Geometry: final body of the model. Coordinates: model frame, mm. A direction names the side the tool comes from. Coordinates: 2 decimals unless noted, no trailing zeros. Loops run counter-clockwise (first coordinate to the right, second up) from the corner with the lowest first, then second, coordinate; pieces in that order, holes last. Notation, with made-up numbers: (30.5, -17) -> (46.5, -17) arc R28 cw to (46.5, 7) -> close; hole circle Ø7 at (-29.75, -38.5). An arc over 180 degrees is marked (long way). One line per item, written item: value. Start each with the question number.
from build123d import *

# Parameters (mm, degrees)
F1_DEPTH      = 19.05
F0_R          = 1.9939
F2_DEPTH      = 2.54
F3_W          = 2.54
F3_H          = 1.905
F4_DEPTH      = 8.89
F5_W          = 2.54
F5_H          = 1.905
F6_DEPTH      = 11.43
F7_W          = 2.54
F7_H          = 2.54
F8_W          = 2.54
F8_H          = 2.54
F9_DEPTH      = 10.16
F10_W         = 2.54
F10_H         = 2.54
F11_DEPTH     = 11.43
F12_T1_DEPTH  = 9.525
F12_T3_DEPTH  = 14.605
F12_T5_DEPTH  = 26.035
F12_T7_DEPTH  = 9.525
F12_T9_DEPTH  = 4.445
F12_T11_DEPTH = 19.685
F12_T13_DEPTH = 22.225
F12_T15_DEPTH = 8.89
F12_T17_DEPTH = 8.89
F12_T19_DEPTH = 8.89
F12_S23_W     = 1.27
F12_S23_H     = 1.27
F12_T24_DEPTH = 1.27
F12_S29_W     = 1.27
F12_S29_H     = 1.27
F12_T30_DEPTH = 1.27


# Not quite as in the source:
# - a fillet or chamfer that OpenCascade refuses, or shapes differently, is made with other operations: its cross-section is extruded or revolved along the edge and cut away or added


with BuildPart() as f1:
    # F0 (on Front) → F1 (new body)
    with BuildSketch(Plane.XZ):
        Polygon((-23.2056408978, -6.35), (-23.2056408978, 0), (-25.7456408978, 0), (-25.7456408978, -8.89), (-9.8706408978, -8.89), (-9.8706408978, 0), (-12.4106408978, 0), (-12.4106408978, -6.35), align=None)
    extrude(amount=F1_DEPTH)

    # F0 (on Front) → F2 (join)
    with BuildSketch(Plane.XZ):
        Polygon((-25.7456408978, -8.89), (-25.7456408978, 0), (-32.0956408978, 0), (-32.0956408978, -12.7), (-3.5206408978, -12.7), (-3.5206408978, 0), (-9.8706408978, 0), (-9.8706408978, -8.89), align=None)
        Polygon((-28.6261399051, -11.2280230969), (-28.955778145, -11.2280230969), (-29.2968038878, -10.3571788012), (-30.3941995557, -10.3571788012), (-30.7310299027, -11.2280230969), (-31.0534760356, -11.2280230969), (-29.9710639241, -8.4782408335), (-29.7031579363, -8.4782408335), align=None, mode=Mode.SUBTRACT)
        with Locations((-28.2856408978, -3.81)):
            Circle(F0_R, mode=Mode.SUBTRACT)
        with Locations((-7.3306408978, -3.81)):
            Circle(F0_R, mode=Mode.SUBTRACT)
    extrude(amount=F2_DEPTH)

    # F3 (on face) → F4 (join)
    with BuildSketch(Plane.XZ.offset(19.05)):
        with Locations((-11.1406408978, -3.4925)):
            Rectangle(F3_W, F3_H)
        with Locations((-24.4756408978, -3.4925)):
            Rectangle(F3_W, F3_H)
    extrude(amount=F4_DEPTH)

    # F5 (on face) → F6 (join)
    with BuildSketch(Plane(origin=(-12.4106408978, 0, 0), x_dir=(0, -1, 0), z_dir=(-1, 0, 0))):
        with Locations((26.67, -3.4925)):
            Rectangle(F5_W, F5_H)
    extrude(amount=F6_DEPTH)

    # F7 (on face) + F8 (on face) → F9 (join)
    with BuildSketch(Plane.XY):
        with Locations((-24.4756408978, -11.43)):
            Rectangle(F7_W, F7_H)
    with BuildSketch(Plane.XY):
        with Locations((-11.1406408978, -11.43)):
            Rectangle(F8_W, F8_H)
    extrude(amount=F9_DEPTH)

    # F10 (on face) → F11 (join)
    with BuildSketch(Plane.YZ.offset(-23.2056408978)):
        with Locations((-11.43, 8.89)):
            Rectangle(F10_W, F10_H)
    extrude(amount=F11_DEPTH)

    # F12: fillet of radius 1.27 on 18 edges, made by hand

    # F12_s2 → F12_t1 (cut)
    with BuildSketch(Plane.YZ.offset(-35.2706408978)):
        with BuildLine():
            ThreePointArc((-1.27, 0), (-2.1680256121, -0.3719743879), (-2.54, -1.27))
            Line((-2.54, -1.27), (-2.54, 0))
            Line((-2.54, 0), (-1.27, 0))
        make_face()
    extrude(amount=F12_T1_DEPTH, mode=Mode.SUBTRACT)

    # F12_s4 → F12_t3 (cut)
    with BuildSketch(Plane.XY.offset(-11.43)):
        with BuildLine():
            ThreePointArc((-32.0956408978, -1.27), (-31.7236665099, -2.1680256121), (-30.8256408978, -2.54))
            Line((-30.8256408978, -2.54), (-32.0956408978, -2.54))
            Line((-32.0956408978, -2.54), (-32.0956408978, -1.27))
        make_face()
        with BuildLine():
            ThreePointArc((-3.5206408978, -1.27), (-3.8926152856, -2.1680256121), (-4.7906408978, -2.54))
            Line((-4.7906408978, -2.54), (-3.5206408978, -2.54))
            Line((-3.5206408978, -2.54), (-3.5206408978, -1.27))
        make_face()
    extrude(amount=F12_T3_DEPTH, mode=Mode.SUBTRACT)

    # F12_s6 → F12_t5 (cut)
    with BuildSketch(Plane.YZ.offset(-30.8256408978)):
        with BuildLine():
            ThreePointArc((-1.27, -12.7), (-2.1680256121, -12.3280256121), (-2.54, -11.43))
            Line((-2.54, -11.43), (-2.54, -12.7))
            Line((-2.54, -12.7), (-1.27, -12.7))
        make_face()
    extrude(amount=F12_T5_DEPTH, mode=Mode.SUBTRACT)

    # F12_s8 → F12_t7 (cut)
    with BuildSketch(Plane.YZ.offset(-9.8706408978)):
        with BuildLine():
            ThreePointArc((-1.27, 0), (-2.1680256121, -0.3719743879), (-2.54, -1.27))
            Line((-2.54, -1.27), (-2.54, 0))
            Line((-2.54, 0), (-1.27, 0))
        make_face()
    extrude(amount=F12_T7_DEPTH, mode=Mode.SUBTRACT)

    # F12_s10 → F12_t9 (cut)
    with BuildSketch(Plane.XZ.offset(-3.175)):
        with BuildLine():
            ThreePointArc((-4.7906408978, -12.7), (-3.8926152856, -12.3280256121), (-3.5206408978, -11.43))
            Line((-3.5206408978, -11.43), (-3.5206408978, -12.7))
            Line((-3.5206408978, -12.7), (-4.7906408978, -12.7))
        make_face()
        with BuildLine():
            ThreePointArc((-32.0956408978, -11.43), (-31.7236665099, -12.3280256121), (-30.8256408978, -12.7))
            Line((-30.8256408978, -12.7), (-32.0956408978, -12.7))
            Line((-32.0956408978, -12.7), (-32.0956408978, -11.43))
        make_face()
    extrude(amount=F12_T9_DEPTH, mode=Mode.SUBTRACT)

    # F12_s12 → F12_t11 (cut)
    with BuildSketch(Plane.XZ.offset(2.54)):
        with BuildLine():
            ThreePointArc((-9.8706408978, -7.62), (-10.2426152856, -8.5180256121), (-11.1406408978, -8.89))
            Line((-11.1406408978, -8.89), (-9.8706408978, -8.89))
            Line((-9.8706408978, -8.89), (-9.8706408978, -7.62))
        make_face()
        with BuildLine():
            ThreePointArc((-25.7456408978, -7.62), (-25.3736665099, -8.5180256121), (-24.4756408978, -8.89))
            Line((-24.4756408978, -8.89), (-25.7456408978, -8.89))
            Line((-25.7456408978, -8.89), (-25.7456408978, -7.62))
        make_face()
    extrude(amount=F12_T11_DEPTH, mode=Mode.SUBTRACT)

    # F12_s14 → F12_t13 (cut)
    with BuildSketch(Plane.YZ.offset(-28.9206408978)):
        with BuildLine():
            ThreePointArc((-26.67, -2.54), (-27.5680256121, -2.9119743879), (-27.94, -3.81))
            Line((-27.94, -3.81), (-27.94, -2.54))
            Line((-27.94, -2.54), (-26.67, -2.54))
        make_face()
        with BuildLine():
            ThreePointArc((-19.05, -7.62), (-18.6780256121, -8.5180256121), (-17.78, -8.89))
            Line((-17.78, -8.89), (-19.05, -8.89))
            Line((-19.05, -8.89), (-19.05, -7.62))
        make_face()
        with BuildLine():
            ThreePointArc((-27.94, -3.175), (-27.5680256121, -4.0730256121), (-26.67, -4.445))
            Line((-26.67, -4.445), (-27.94, -4.445))
            Line((-27.94, -4.445), (-27.94, -3.175))
        make_face()
        with BuildLine():
            ThreePointArc((-11.43, 10.16), (-12.3280256121, 9.7880256121), (-12.7, 8.89))
            Line((-12.7, 8.89), (-12.7, 10.16))
            Line((-12.7, 10.16), (-11.43, 10.16))
        make_face()
        with BuildLine():
            ThreePointArc((-10.16, 8.89), (-10.5319743879, 9.7880256121), (-11.43, 10.16))
            Line((-11.43, 10.16), (-10.16, 10.16))
            Line((-10.16, 10.16), (-10.16, 8.89))
        make_face()
    extrude(amount=F12_T13_DEPTH, mode=Mode.SUBTRACT)

    # F12_s16 → F12_t15 (cut)
    with BuildSketch(Plane.YZ.offset(-28.9206408978)):
        with BuildLine():
            ThreePointArc((-19.05, -1.27), (-18.6780256121, -0.3719743879), (-17.78, 0))
            Line((-17.78, 0), (-19.05, 0))
            Line((-19.05, 0), (-19.05, -1.27))
        make_face()
    extrude(amount=F12_T15_DEPTH, mode=Mode.SUBTRACT)

    # F12_s18 → F12_t17 (cut)
    with BuildSketch(Plane.YZ.offset(-15.5856408978)):
        with BuildLine():
            ThreePointArc((-17.78, 0), (-18.6780256121, -0.3719743879), (-19.05, -1.27))
            Line((-19.05, -1.27), (-19.05, 0))
            Line((-19.05, 0), (-17.78, 0))
        make_face()
    extrude(amount=F12_T17_DEPTH, mode=Mode.SUBTRACT)

    # F12_s20 → F12_t19 (cut)
    with BuildSketch(Plane.XZ.offset(6.985)):
        with BuildLine():
            ThreePointArc((-25.7456408978, 8.89), (-25.3736665099, 9.7880256121), (-24.4756408978, 10.16))
            Line((-24.4756408978, 10.16), (-25.7456408978, 10.16))
            Line((-25.7456408978, 10.16), (-25.7456408978, 8.89))
        make_face()
        with BuildLine():
            ThreePointArc((-9.8706408978, 8.89), (-10.2426152856, 9.7880256121), (-11.1406408978, 10.16))
            Line((-11.1406408978, 10.16), (-9.8706408978, 10.16))
            Line((-9.8706408978, 10.16), (-9.8706408978, 8.89))
        make_face()
    extrude(amount=F12_T19_DEPTH, mode=Mode.SUBTRACT)


with BuildPart() as f12_tool22:
    # F12_s23 → F12_t24 (new body)
    with BuildSketch(Plane.YZ.offset(-30.8256408978)):
        with Locations((-1.905, -12.065)):
            Rectangle(F12_S23_W, F12_S23_H)
    extrude(amount=-F12_T24_DEPTH)

    # F12_s25 → F12_t26 (revolve, cut)
    with BuildSketch(Plane(origin=(-30.8256408978, -1.27, -11.43), x_dir=(0, 0.7071067812, 0.7071067812), z_dir=(0, -0.7071067812, 0.7071067812))):
        with BuildLine():
            ThreePointArc((0, -1.27), (1.27, 0), (0, 1.27))
            Line((0, 1.27), (0, -1.27))
        make_face()
    revolve(axis=Axis((-30.8256408978, -1.27, -11.43), (-1, 0, 0)), mode=Mode.SUBTRACT)


with BuildPart() as f1_1:
    add(f1.part)

    # F12_t21: cut F12_tool22
    add(f12_tool22.part, mode=Mode.SUBTRACT)


with BuildPart() as f12_tool28:
    # F12_s29 → F12_t30 (new body)
    with BuildSketch(Plane.YZ.offset(-4.7906408978)):
        with Locations((-1.905, -12.065)):
            Rectangle(F12_S29_W, F12_S29_H)
    extrude(amount=F12_T30_DEPTH)

    # F12_s31 → F12_t32 (revolve, cut)
    with BuildSketch(Plane(origin=(-4.7906408978, -1.27, -11.43), x_dir=(0, 0.7071067812, 0.7071067812), z_dir=(0, 0.7071067812, -0.7071067812))):
        with BuildLine():
            ThreePointArc((0, -1.27), (1.27, 0), (0, 1.27))
            Line((0, 1.27), (0, -1.27))
        make_face()
    revolve(axis=Axis((-4.7906408978, -1.27, -11.43), (1, 0, 0)), mode=Mode.SUBTRACT)


with BuildPart() as f1_2:
    add(f1_1.part)

    # F12_t27: cut F12_tool28
    add(f12_tool28.part, mode=Mode.SUBTRACT)


solid = f1_2.part
1. Section A-A on z = 2.75. Return the cut outline in (x, y), plus the area to 3 significant figures.
2. Pin query (flat end, axial travel): pin 1 Ø2.5 at (x, z) = (-15.5, -6.5) entering from -Y; pin 2 Ø7 at (x, y) = (-7.5, -5) entering from +Z; pin 3 Ø4 at (x, y) = (-7, -19.5) entering from +Z (3 decimals); pin 4 Ø2 at (x, y) = (-24, -16.5) entering from -Z. Return the tip coordinate at first contact, or that it passes through.
3. Draft query along Z for faces 4 (the face through (-16, -26, -2.54)), 5 (the face through (-3.903, -0.626, -12.338)), 6 (the face through (-18, -25.4, -4)), 7 (the face through (-29.172, -1.252, -9.834)). Return one class per face: released by +Z, released by -Z, zero draft, split by the parting line, or undercut.
4. Section C-C on y = -14.25. Return the cut outline in (x, z).
5. Line query: L1, parallel to X at y = -11.25, z = 6.25; L2, parallel to Y at x = -8.25, z = -9.5; L3, parallel to Y at x = -18.25, z = -7. Output: solid intervals per line, ascending. Write a range as [from, to].
6. Section B-B on x = -18. Count the separate pieces of the cut face and the enclosed holes in it, plus the area to 3 significant figures.
7. Set-up query: faces 1 (the face through (-23.206, -13, -3)), 2 (the face through (-29.124, -1.252, -10.799)), 3 (the face through (-10.233, -10.679, -8.508)). Return all of +Z, -Z, +X, -X, +Y, -Y with unobstructed straight access to the full face (end or side cutting, diameter ignored); none if empty.
8. Section D-D on y = -11. Return the cut outline in (x, z), plus the area to 3 significant figures.
Checks:
1. outline: (-25.75, -12.7) -> (-23.21, -12.7) -> (-23.21, -10.16) -> (-25.75, -10.16) -> close; (-12.41, -12.7) -> (-9.87, -12.7) -> (-9.87, -10.16) -> (-12.41, -10.16) -> close
1. area: 12.9 mm²
2. pin 1: y = -19.05
2. pin 2: z = 0
2. pin 3: through
2. pin 4: z = -8.89
3. face 4: released by +Z
3. face 5: released by -Z
3. face 6: zero draft
3. face 7: undercut
4. outline: (-25.75, -7.62) arc R1.27 ccw to (-24.48, -8.89) -> (-11.14, -8.89) arc R1.27 ccw to (-9.87, -7.62) -> (-9.87, 0) -> (-12.41, 0) -> (-12.41, -6.35) -> (-23.21, -6.35) -> (-23.21, 0) -> (-25.75, 0) -> close
5. L1: [-25.75, -23.21], [-12.41, -9.87]
5. L2: [-2.54, 0]
5. L3: [-19.05, 0]
6. separate pieces: 3
6. enclosed holes: 0
6. area: 67.3 mm²
7. face 1: +Y
7. face 2: +Y, -Y
7. face 3: -Z, +X, -Y
8. outline: (-25.75, -7.62) arc R1.27 ccw to (-24.48, -8.89) -> (-11.14, -8.89) arc R1.27 ccw to (-9.87, -7.62) -> (-9.87, 8.89) arc R1.27 ccw to (-10.71, 10.08) -> (-24.91, 10.08) arc R1.27 ccw to (-25.75, 8.89) -> close; hole (-23.21, -6.35) -> (-12.41, -6.35) -> (-12.41, 7.62) -> (-23.21, 7.62) -> close
8. area: 149 mm²
